Design review of the part built by this model. Coordinates are the model's own, in mm. A direction names the side the tool comes from. Round coordinates to 2 decimals unless told otherwise and drop trailing zeros. Order: outer loops, then holes, each group sorted by start corner. A loop starts at its lowest first (then second) coordinate and runs counter-clockwise, first axis right, second up. Notation, with made-up numbers: M 44.5,-1.75 L 95.5,-1.75 A16 ccw 95.5,5.25 Z; hole C 20.5,-1.5 d4. An arc over 180 degrees is marked long. Use a Markdown table: item, result. Add a question column.
(1) For pin 1 (4 mm diameter, centred on x = -7, y = 19.5, fed in from +Z); pin 2 (1.9 mm diameter, centred on x = -16, y = 4, fed in from -Z); pin 3 (1 mm diameter, centred on x = 1.5, z = 9, fed in from -Y); pin 4 (5 mm diameter, centred on x = 12, y = 8, fed in from +Z), all flat-tipped, find the tip position at first contact; note any pin that passes through.
(2) Machinability: for faces 5 (the face through (1.42, 4.93, -18.46)), 6 (the face through (14.38, 4.93, -8.91)), 7 (the face through (8, 10, -9)), which of the approach directions +Z, -Z, +X, -X, +Y, -Y give a long, thin tool a straight path to every point of the face, cutting with its end or side? Answer none if there is none.
(3) Take a section at B-B (y = 6). Write out the cut boundary in (x, z) (3 decimals).
(4) To check wall thickness, follow probe 1 along X at (y, z) = (17.75, 0); probe 2 along X at (y, z) = (13.5, -4.5); probe 3 along Y at (x, z) = (4.5, -12). State the ranges of each line that lie inside material, in increasing order. Write a range as from..to.
(5) The part is to be moulded in two halves that separate along X. For faces 1 (the face through (9.7, 19.86, 6.18)), 2 (the face through (15.3, 4.9, 10.5)), 3 (the face through (7.03, 4.93, 11.94)), 4 (the face through (8.074, 4.843, 14.209)), say which applies: released by +X, released by -X, zero draft, split by the parting line, or undercut.
(6) Take a section at C-C (y = 10.5). Write out the cut boundary in (x, z).
(7) Take a section at D-D (x = 10.5). Count the separate pieces of the cut face and the enclosed holes in it, then the cut area to 3 significant figures.
(8) Take a section at A-A (z = 0). Write out the cut boundary in (x, y), then the cut area to 3 significant figures.
```python
from build123d import *

# Parameters (mm, degrees)
SKETCH1_R           = 11.5
BOSS_EXTRUDE1_DEPTH = 30
SKETCH4_R           = 11.5
CUT_EXTRUDE1_DEPTH  = 10
SKETCH5_R           = 1
CUT_EXTRUDE2_DEPTH  = 46.027075188
SKETCH6_R           = 1
CUT_EXTRUDE3_DEPTH  = 46.928613086
SKETCH7_R           = 1
CUT_EXTRUDE4_DEPTH  = 46.928613086


with BuildPart() as part:
    # Sketch1 → Boss-Extrude1 (new body)
    with BuildSketch(Plane(origin=(0, 0, 0), x_dir=(1, 0, 0), z_dir=(0, 1, 0))):
        Polygon((0, 20.5), (-17.753520778, 10.25), (-17.753520778, -10.25), (0, -20.5), (17.753520778, -10.25), (17.753520778, 10.25), align=None)
        with Locations(Location((0, 0, 0), (0, 0, 270))):
            Circle(SKETCH1_R, mode=Mode.SUBTRACT)
    extrude(amount=BOSS_EXTRUDE1_DEPTH)

    # Sketch2 → Cut-Revolve1 (revolve, cut)
    with BuildSketch(Plane.XY, mode=Mode.PRIVATE) as cut_revolve1_sk:
        Polygon((20.5, 13.897411558), (13, 30), (0, 30), (0, 31.097791256), (25.351389146, 31.097791256), (24.973358823, 13.897411558), align=None)
    revolve(cut_revolve1_sk.sketch.rotate(Axis((0, 30, 0), (0, -1, 0)), 90), axis=Axis((0, 30, 0), (0, -1, 0)), mode=Mode.SUBTRACT)

    # Sketch4 → Cut-Extrude1 (cut)
    with BuildSketch(Plane.XZ):
        Polygon((-13.856406461, -8), (-17.753520778, -8), (-17.753520778, -10.25), (0, -20.5), (1.948557159, -19.375), (0, -16), (13.856406461, -8), (15.804963619, -11.375), (17.753520778, -10.25), (17.753520778, 10.25), (15.804963619, 11.375), (13.856406461, 8), (0, 16), (1.948557159, 19.375), (0, 20.5), (-17.753520778, 10.25), (-17.753520778, 8), (-13.856406461, 8), align=None)
        with Locations(Location((0, 0, 0), (0, 0, 270))):
            Circle(SKETCH4_R, mode=Mode.SUBTRACT)
    extrude(amount=-CUT_EXTRUDE1_DEPTH, mode=Mode.SUBTRACT)

    # Sketch5 → Cut-Extrude2 (cut, through all)
    with BuildSketch(Plane.XY.offset(8)):
        with Locations((-15.804963619, 4)):
            Circle(SKETCH5_R)
    extrude(amount=-CUT_EXTRUDE2_DEPTH, mode=Mode.SUBTRACT)

    # Sketch6 → Cut-Extrude3 (cut, through all)
    with BuildSketch(Plane(origin=(-6.92820323, 0, 4), x_dir=(0.5000000000000042, 0, 0.8660254037844363), z_dir=(-0.8660254037844362, 0, 0.5000000000000041))):
        with Locations((15.804963619, 4)):
            Circle(SKETCH6_R)
    extrude(amount=-CUT_EXTRUDE3_DEPTH, mode=Mode.SUBTRACT)

    # Sketch7 → Cut-Extrude4 (cut, through all)
    with BuildSketch(Plane(origin=(6.92820323, 0, 4), x_dir=(0.4999999999999912, 0, -0.8660254037844437), z_dir=(0.8660254037844437, 0, 0.4999999999999912))):
        with Locations((15.804963619, 4)):
            Circle(SKETCH7_R)
    extrude(amount=-CUT_EXTRUDE4_DEPTH, mode=Mode.SUBTRACT)


solid = part.part
```
Verdict:
| question | item | result |
|---|---|---|
| 1 | pin 1 | stops at z = 17.52 |
| 1 | pin 2 | stops at z = -8 |
| 1 | pin 3 | passes through |
| 1 | pin 4 | stops at z = 15.02 |
| 2 | face 5 | -Z, -X, -Y |
| 2 | face 6 | +X, -Y |
| 2 | face 7 | -Y |
| 3 | outline | M -17.754,-8 L -13.856,-8 L -13.856,8 L -17.754,8 Z; M 0,-16 L 1.949,-19.375 L 15.805,-11.375 L 13.856,-8 Z; M 0,16 L 13.856,8 L 15.805,11.375 L 1.949,19.375 Z |
| 4 | probe 1 | x = -17.75..-11.5, 11.5..17.75 |
| 4 | probe 2 | x = -17.75..-10.58, 10.58..17.75 |
| 4 | probe 3 | y = 10..30 |
| 5 | face 1 | undercut |
| 5 | face 2 | released by +X |
| 5 | face 3 | released by -X |
| 5 | face 4 | undercut |
| 6 | outline | M -17.75,-10.25 L 0,-20.5 L 17.75,-10.25 L 17.75,10.25 L 0,20.5 L -17.75,10.25 Z; hole C 0,0 d23 |
| 7 | separate pieces | 2 |
| 7 | enclosed holes | 2 |
| 7 | area | 406 mm^2 |
| 8 | outline | M -17.75,0 L -13.86,0 L -13.86,10 L -11.5,10 L -11.5,30 L -13,30 L -17.75,19.79 Z; M 11.5,10 L 17.75,10 L 17.75,19.79 L 13,30 L 11.5,30 Z; hole C -15.8,4 d2 |
| 8 | area | 237 mm^2 |
